For this review, take the finished solid that the model builds, in its own axes (mm). Round coordinates to 2 decimals unless told otherwise and drop trailing zeros. Write each loop counter-clockwise with the first axis right and the second up, starting at its lowest first coordinate (ties: lowest second). Pieces come first, ordered by that corner, then holes. Notation, with made-up numbers: (-23.5, -23.75) - (-10.5, -23.75) arc R28 cw to (-10.5, 14.25) - close; hole circle Ø8 at (-6, -16). An arc over 180 degrees is marked (long way). One line per item, written item: value. Start each with the question number.
Q1. Add section B-B on z = -25.4. Write out the cut boundary in (x, y), and give its area (3 significant figures).
Q2. Add section C-C on x = 20. Write out the cut boundary in (y, z) (3 decimals), and give its area (3 significant figures).
Q3. For probe 1 along X at (y, z) = (5, -25.4); probe 2 along Y at (x, z) = (8.25, -42.9) (3 decimals); probe 3 along X at (y, z) = (4.25, -5), list the stretches that pass through material, from the lowest coordinate up.
Q4. Add section A-A on x = 165. Write out the cut boundary in (y, z).
Q5. Clearance check with a flat-ended pin moving along its axis: pin 1 Ø5 at (x, z) = (74, -25.4) entering from +Y. State where the tip first meets the part, or that it passes through.
```python
from build123d import *

# Parameters (mm, degrees)
SKETCH1_W                 = 170
SKETCH1_H                 = 50.8
SKETCH1_R                 = 2.25
BOSS_EXTRUDE1_DEPTH       = 6.35
CHAMFER1_SIZE             = 15
M4X0_7_TAPPED_HOLE1_D     = 3.3
M4X0_7_TAPPED_HOLE1_DEPTH = 25.4
M4X0_7_TAPPED_HOLE1_TIP   = 0.991420021


with BuildPart() as part:
    # Sketch1 → Boss-Extrude1 (new body)
    with BuildSketch(Plane(origin=(0, 0, 0), x_dir=(1, 0, 0), z_dir=(0, 1, 0))):
        with Locations((85, 25.4)):
            Rectangle(SKETCH1_W, SKETCH1_H)
        with Locations(Location((165, 25.4, 0), (0, 0, 270))):
            Circle(SKETCH1_R, mode=Mode.SUBTRACT)
        with Locations(Location((73.999999882, 25.4, 0), (0, 0, 270))):
            Circle(SKETCH1_R, mode=Mode.SUBTRACT)
        with Locations(Location((41.619, 44.45, 0), (0, 0, 270))):
            Circle(SKETCH1_R, mode=Mode.SUBTRACT)
        with Locations(Location((41.619, 6.35, 0), (0, 0, 270))):
            Circle(SKETCH1_R, mode=Mode.SUBTRACT)
    extrude(amount=BOSS_EXTRUDE1_DEPTH)

    # Chamfer1
    chamfer1_edges = [part.edges().sort_by_distance(p)[0] for p in [
        (170, 3.175, -50.8),
        (170, 3.175, 0),
    ]]
    chamfer(chamfer1_edges, length=CHAMFER1_SIZE)

    # M4x0.7 Tapped Hole1
    with Locations(Plane.ZY):
        with Locations((-42.9, 3.175), (-7.9, 3.175)):
            Hole(M4X0_7_TAPPED_HOLE1_D / 2, depth=M4X0_7_TAPPED_HOLE1_DEPTH)
            with Locations((0, 0, -(M4X0_7_TAPPED_HOLE1_DEPTH + M4X0_7_TAPPED_HOLE1_TIP / 2))):  # 118° drill point
                Cone(0, M4X0_7_TAPPED_HOLE1_D / 2, M4X0_7_TAPPED_HOLE1_TIP, mode=Mode.SUBTRACT)


solid = part.part
```
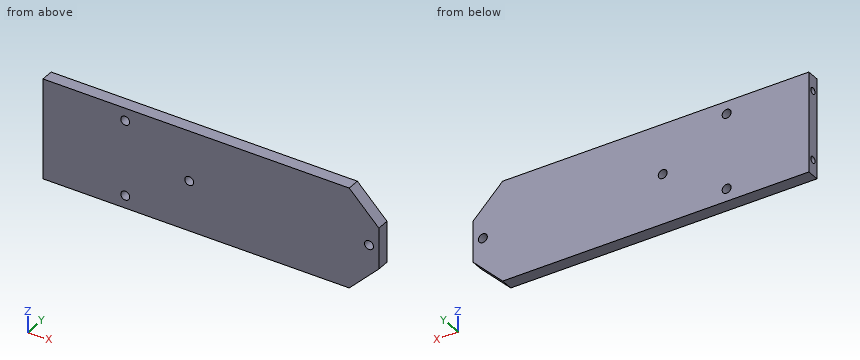
Result set:
1. outline: (0, 0) - (71.75, 0) - (71.75, 6.35) - (0, 6.35) - close; (76.25, 0) - (162.75, 0) - (162.75, 6.35) - (76.25, 6.35) - close; (167.25, 0) - (170, 0) - (170, 6.35) - (167.25, 6.35) - close
1. area: 1,020 mm^2
2. outline: (0, -50.8) - (6.35, -50.8) - (6.35, 0) - (0, 0) - close; hole circle Ø3.3 at (3.175, -42.9); hole circle Ø3.3 at (3.175, -7.9)
2. area: 305 mm^2
3. probe 1: x = 0 to 71.75, 76.25 to 162.75, 167.25 to 170
3. probe 2: y = 0 to 1.525, 4.825 to 6.35
3. probe 3: x = 0 to 39.82, 43.42 to 160
4. outline: (0, -40.8) - (6.35, -40.8) - (6.35, -27.65) - (0, -27.65) - close; (0, -23.15) - (6.35, -23.15) - (6.35, -10) - (0, -10) - close
5. pin 1: stops at y = 6.35
